The listing builds one solid part. Answer for the finished solid, in the listing's coordinates (mm). Face numbers are marked on the shaded views. A direction names the side the tool comes from. Round coordinates to 2 decimals unless told otherwise and drop trailing zeros. Write each loop counter-clockwise with the first axis right and the second up, starting at its lowest first coordinate (ties: lowest second). Pieces come first, ordered by that corner, then holes. Notation, with made-up numbers: M -9,46 L 29,46 A12 ccw 29,68 Z; hole C -34.75,-31 d8. An arc over 180 degrees is marked long. Put each result on its own line as item: value. Start each with the question number.
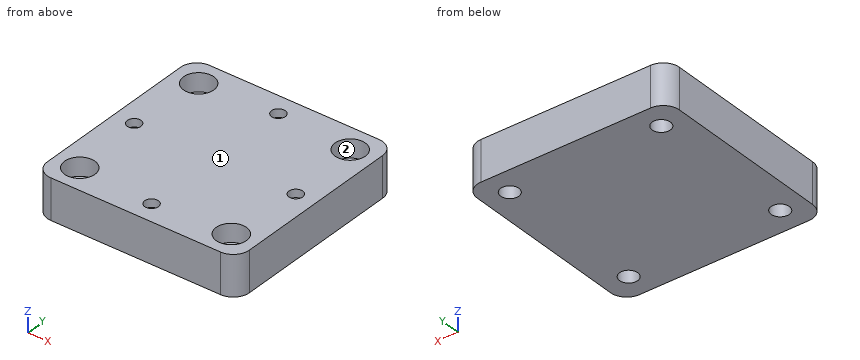
Autodesk Fusion 360 part; units mm, degrees
sketch "Sketch1" plane through (0, 0, 0) normal (0, 0, 1) x (1, 0, 0)
  line L0 (0, 0) -> (-50, 0)
  line L1 (-50, 0) -> (-50, 50)
  line L2 (-50, 50) -> (0, 50)
  line L3 (0, 50) -> (0, 0)
  dimension "d1" = 50
  dimension "d2" = 50
extrude "Extrude1" add sketch "Sketch1" along normal blind 10
sketch "Sketch2" plane through (0, 0, 10) normal (0, 0, 1) x (-1, 0, 0)
  line L0 (0, -50) -> (50, -50)
  line L1 (50, -50) -> (50, 0)
  line L2 (50, 0) -> (0, 0)
  line L3 (0, 0) -> (0, -50)
  line L4 (50, 0) -> (43.75, 0)
  line L5 (43.75, 0) -> (43.75, -6.25)
  line L6 (43.75, -6.25) -> (50, -6.25)
  line L7 (50, -6.25) -> (50, 0)
  line L8 (50, -50) -> (43.75, -50)
  line L9 (43.75, -50) -> (43.75, -43.75)
  line L10 (43.75, -43.75) -> (50, -43.75)
  line L11 (50, -43.75) -> (50, -50)
  line L12 (0, -50) -> (6.25, -50)
  line L13 (6.25, -50) -> (6.25, -43.75)
  line L14 (6.25, -43.75) -> (0, -43.75)
  line L15 (0, -43.75) -> (0, -50)
  line L16 (0, 0) -> (6.25, 0)
  line L17 (6.25, 0) -> (6.25, -6.25)
  line L18 (6.25, -6.25) -> (0, -6.25)
  line L19 (0, -6.25) -> (0, 0)
  circle A0 centre (43.75, -43.75) radius 3.75
  circle A1 centre (6.25, -43.75) radius 3.75
  circle A2 centre (43.75, -6.25) radius 3.75
  circle A3 centre (6.25, -6.25) radius 3.75
  dimension "d5" = 6.25
  dimension "d6" = 6.25
  dimension "d7" = 6.25
  dimension "d8" = 6.25
  dimension "d9" = 6.25
  dimension "d10" = 6.25
  dimension "d11" = 6.25
  dimension "d12" = 6.25
  dimension "d13" = 7.5
  dimension "d14" = 7.5
  dimension "d15" = 7.5
  dimension "d16" = 7.5
extrude "Extrude2" cut sketch "Sketch2" against normal blind 4.5 contours L13 L14 A1 | L13 L14 A1 | L9 L10 A0 | L9 L10 A0 | L17 L18 A3 | L17 L18 A3 | L5 L6 A2 | L5 L6 A2
sketch "Sketch3" plane through (0, 0, 5.5) normal (0, 0, 1) x (-1, 0, 0)
  circle A0 centre (43.75, -43.75) radius 3.75
  circle A1 centre (43.75, -43.75) radius 2.25
  dimension "d19" = 4.5
extrude "Extrude3" cut sketch "Sketch3" against normal blind 10 contours A1
sketch "Sketch4" plane through (0, 0, 5.5) normal (0, 0, 1) x (-1, 0, 0)
  circle A0 centre (6.25, -43.75) radius 3.75
  circle A1 centre (6.25, -43.75) radius 2.25
  dimension "d22" = 4.5
extrude "Extrude4" cut sketch "Sketch4" against normal blind 10 contours A1
sketch "Sketch5" plane through (0, 0, 5.5) normal (0, 0, 1) x (-1, 0, 0)
  circle A0 centre (43.75, -6.25) radius 3.75
  circle A1 centre (43.75, -6.25) radius 2.25
  dimension "d25" = 4.5
extrude "Extrude5" cut sketch "Sketch5" against normal blind 10 contours A1
sketch "Sketch6" plane through (0, 0, 5.5) normal (0, 0, 1) x (-1, 0, 0)
  circle A0 centre (6.25, -6.25) radius 3.75
  circle A1 centre (6.25, -6.25) radius 2.25
  dimension "d28" = 4.5
extrude "Extrude6" cut sketch "Sketch6" against normal blind 10 contours A1
sketch "Sketch7" plane through (0, 0, 10) normal (0, 0, 1) x (-1, 0, 0)
  circle A0 centre (6.25, -43.75) radius 3.75
  circle A1 centre (6.25, -6.25) radius 3.75
  circle A2 centre (43.75, -43.75) radius 3.75
  circle A3 centre (43.75, -6.25) radius 3.75
  line L0 (0, -50) -> (50, -50)
  line L1 (50, -50) -> (50, 0)
  line L2 (50, 0) -> (0, 0)
  line L3 (0, 0) -> (0, -50)
  line L4 (50, 0) -> (37.5, 0)
  line L5 (37.5, 0) -> (37.5, -12.5)
  line L6 (37.5, -12.5) -> (50, -12.5)
  line L7 (50, -12.5) -> (50, 0)
  line L8 (50, -50) -> (37.5, -50)
  line L9 (37.5, -50) -> (37.5, -37.5)
  line L10 (37.5, -37.5) -> (50, -37.5)
  line L11 (50, -37.5) -> (50, -50)
  line L12 (0, -50) -> (12.5, -50)
  line L13 (12.5, -50) -> (12.5, -37.5)
  line L14 (12.5, -37.5) -> (0, -37.5)
  line L15 (0, -37.5) -> (0, -50)
  line L16 (0, 0) -> (12.5, 0)
  line L17 (12.5, 0) -> (12.5, -12.5)
  line L18 (12.5, -12.5) -> (0, -12.5)
  line L19 (0, -12.5) -> (0, 0)
  line L20 (37.5, -12.5) -> (35.5, -12.5)
  line L21 (35.5, -12.5) -> (35.5, -14.5)
  line L22 (35.5, -14.5) -> (37.5, -14.5)
  line L23 (37.5, -14.5) -> (37.5, -12.5)
  line L24 (37.5, -37.5) -> (35.5, -37.5)
  line L25 (35.5, -37.5) -> (35.5, -35.5)
  line L26 (35.5, -35.5) -> (37.5, -35.5)
  line L27 (37.5, -35.5) -> (37.5, -37.5)
  line L28 (12.5, -37.5) -> (14.5, -37.5)
  line L29 (14.5, -37.5) -> (14.5, -35.5)
  line L30 (14.5, -35.5) -> (12.5, -35.5)
  line L31 (12.5, -35.5) -> (12.5, -37.5)
  line L32 (12.5, -12.5) -> (14.5, -12.5)
  line L33 (14.5, -12.5) -> (14.5, -14.5)
  line L34 (14.5, -14.5) -> (12.5, -14.5)
  line L35 (12.5, -14.5) -> (12.5, -12.5)
  dimension "d31" = 12.5
  dimension "d32" = 12.5
  dimension "d33" = 12.5
  dimension "d34" = 12.5
  dimension "d35" = 12.5
  dimension "d36" = 12.5
  dimension "d37" = 12.5
  dimension "d38" = 12.5
  dimension "d39" = 2
  dimension "d40" = 2
  dimension "d41" = 2
  dimension "d42" = 2
  dimension "d43" = 2
  dimension "d44" = 2
  dimension "d45" = 2
  dimension "d46" = 2
extrude "Extrude7" add sketch "Sketch7" along normal blind 2 contours L24 L25 L26 L27 | L20 L21 L22 L23 | L32 L33 L34 L35 | L28 L29 L30 L31
extrude "Extrude8" cut 4 faces at (-13.1667, 36.1667, 12) (-13.1667, 13.1667, 12) (-36.1667, 13.1667, 12) (-36.8333, 36.8333, 12) along direction (0, 0, -1) blind 2
fillet "Fillet1" radius 4 1 edges at (0, 50, 5)
fillet "Fillet2" radius 4 1 edges at (0, 0, 5)
fillet "Fillet3" radius 4 1 edges at (-50, 50, 5)
fillet "Fillet4" radius 4 1 edges at (-50, 0, 5)
sketch "Sketch8" plane through (0, 0, 10) normal (0, 0, 1) x (-1, 0, 0)
  circle A0 centre (6.25, -43.75) radius 3.75
  circle A1 centre (6.25, -6.25) radius 3.75
  circle A2 centre (43.75, -43.75) radius 3.75
  circle A3 centre (43.75, -6.25) radius 3.75
  arc A4 (50, -4) -> (46, 0) centre (46, -4) ccw
  line L0 (46, 0) -> (4, 0)
  arc A5 (4, 0) -> (0, -4) centre (4, -4) ccw
  line L1 (0, -4) -> (0, -46)
  arc A6 (0, -46) -> (4, -50) centre (4, -46) ccw
  line L2 (4, -50) -> (46, -50)
  arc A7 (46, -50) -> (50, -46) centre (46, -46) ccw
  line L3 (50, -46) -> (50, -4)
  line L4 (0, 0) -> (5, 0)
  line L5 (5, 0) -> (5, -5)
  line L6 (5, -5) -> (0, -5)
  line L7 (0, -5) -> (0, 0)
  line L8 (5, -5) -> (45, -5)
  line L9 (45, -5) -> (45, -45)
  line L10 (45, -45) -> (5, -45)
  line L11 (5, -45) -> (5, -5)
  circle A8 centre (25, -45) radius 1.6
  circle A9 centre (45, -25) radius 1.6
  circle A10 centre (25, -5) radius 1.6
  circle A11 centre (5, -25) radius 1.6
  dimension "d59" = 5
  dimension "d60" = 5
  dimension "d61" = 40
  dimension "d62" = 40
  dimension "d63" = 3.2
  dimension "d64" = 3.2
  dimension "d65" = 3.2
  dimension "d66" = 3.2
extrude "Extrude9" cut sketch "Sketch8" against normal blind 2 contours L11 A11 | L11 A11 | L10 A8 | L10 A8 | L9 A9 | L9 A9 | L8 A10 | L8 A10
sketch "Sketch9" plane through (0, 0, 10) normal (0, 0, 1) x (-1, 0, 0)
  circle A0 centre (25, -45) radius 1.6
  circle A1 centre (5, -25) radius 1.6
  circle A2 centre (45, -25) radius 1.6
  circle A3 centre (25, -5) radius 1.6
  circle A4 centre (6.25, -43.75) radius 3.75
  circle A5 centre (6.25, -6.25) radius 3.75
  circle A6 centre (43.75, -43.75) radius 3.75
  circle A7 centre (43.75, -6.25) radius 3.75
  arc A8 (50, -4) -> (46, 0) centre (46, -4) ccw
  line L0 (46, 0) -> (4, 0)
  arc A9 (4, 0) -> (0, -4) centre (4, -4) ccw
  line L1 (0, -4) -> (0, -46)
  arc A10 (0, -46) -> (4, -50) centre (4, -46) ccw
  line L2 (4, -50) -> (46, -50)
  arc A11 (46, -50) -> (50, -46) centre (46, -46) ccw
  line L3 (50, -46) -> (50, -4)
  circle A12 centre (25, -5) radius 1.7
  dimension "d69" = 3.4
extrude "Extrude10" cut sketch "Sketch9" against normal blind 2 contours A12
sketch "Sketch10" plane through (0, 0, 10) normal (0, 0, 1) x (-1, 0, 0)
  circle A0 centre (25, -5) radius 1.7
  circle A1 centre (25, -45) radius 1.6
  circle A2 centre (5, -25) radius 1.6
  circle A3 centre (45, -25) radius 1.6
  circle A4 centre (6.25, -43.75) radius 3.75
  circle A5 centre (6.25, -6.25) radius 3.75
  circle A6 centre (43.75, -43.75) radius 3.75
  circle A7 centre (43.75, -6.25) radius 3.75
  arc A8 (50, -4) -> (46, 0) centre (46, -4) ccw
  line L0 (46, 0) -> (4, 0)
  arc A9 (4, 0) -> (0, -4) centre (4, -4) ccw
  line L1 (0, -4) -> (0, -46)
  arc A10 (0, -46) -> (4, -50) centre (4, -46) ccw
  line L2 (4, -50) -> (46, -50)
  arc A11 (46, -50) -> (50, -46) centre (46, -46) ccw
  line L3 (50, -46) -> (50, -4)
  circle A12 centre (45, -25) radius 1.7
  dimension "d72" = 3.4
extrude "Extrude11" cut sketch "Sketch10" against normal blind 2 contours A12
sketch "Sketch11" plane through (0, 0, 10) normal (0, 0, 1) x (-1, 0, 0)
  circle A0 centre (45, -25) radius 1.7
  circle A1 centre (25, -5) radius 1.7
  circle A2 centre (25, -45) radius 1.6
  circle A3 centre (5, -25) radius 1.6
  circle A4 centre (6.25, -43.75) radius 3.75
  circle A5 centre (6.25, -6.25) radius 3.75
  circle A6 centre (43.75, -43.75) radius 3.75
  circle A7 centre (43.75, -6.25) radius 3.75
  arc A8 (50, -4) -> (46, 0) centre (46, -4) ccw
  line L0 (46, 0) -> (4, 0)
  arc A9 (4, 0) -> (0, -4) centre (4, -4) ccw
  line L1 (0, -4) -> (0, -46)
  arc A10 (0, -46) -> (4, -50) centre (4, -46) ccw
  line L2 (4, -50) -> (46, -50)
  arc A11 (46, -50) -> (50, -46) centre (46, -46) ccw
  line L3 (50, -46) -> (50, -4)
  circle A12 centre (5, -25) radius 1.7
  dimension "d75" = 3.4
extrude "Extrude12" cut sketch "Sketch11" against normal blind 2 contours A12
sketch "Sketch12" plane through (0, 0, 10) normal (0, 0, 1) x (-1, 0, 0)
  circle A0 centre (5, -25) radius 1.7
  circle A1 centre (45, -25) radius 1.7
  circle A2 centre (25, -5) radius 1.7
  circle A3 centre (25, -45) radius 1.6
  circle A4 centre (6.25, -43.75) radius 3.75
  circle A5 centre (6.25, -6.25) radius 3.75
  circle A6 centre (43.75, -43.75) radius 3.75
  circle A7 centre (43.75, -6.25) radius 3.75
  arc A8 (50, -4) -> (46, 0) centre (46, -4) ccw
  line L0 (46, 0) -> (4, 0)
  arc A9 (4, 0) -> (0, -4) centre (4, -4) ccw
  line L1 (0, -4) -> (0, -46)
  arc A10 (0, -46) -> (4, -50) centre (4, -46) ccw
  line L2 (4, -50) -> (46, -50)
  arc A11 (46, -50) -> (50, -46) centre (46, -46) ccw
  line L3 (50, -46) -> (50, -4)
  circle A12 centre (25, -45) radius 1.7
  dimension "d78" = 3.4
extrude "Extrude13" cut sketch "Sketch12" against normal blind 2 contours A12
Item 1: Flat-ended cylindrical pins translate along their axes: pin 1 (2.5 mm diameter, centred on x = -6.25, y = 43.75, fed in from +Z); pin 2 (1.7 mm diameter, centred on x = -25, y = 5.5, fed in from +Z); pin 3 (7 mm diameter, centred on x = -6.25, y = 6.25, fed in from +Z). Find the tip coordinate at first contact, or state that the pin passes through.
Item 2: Which of the six approach directions +Z, -Z, +X, -X, +Y, -Y give full straight-line access (tool end or side, diameter ignored) to the marked faces 1 and 2?
Item 3: Section B-B (x = -45) is taken. Give the vertices of the cut face in (y, z), and give its area (3 significant figures).
Item 4: Consider line 1 along Y through (x, z) = (-25, 9); line 2 along X through (y, z) = (25, 9.3); line 3 along Y through (x, z) = (-43.75, 1.7). Determine where each line is inside the solid, lowest interval first. Write a range as [from, to].
Item 5: Section A-A (z = 6.5) is taken. Give the vertices of the cut face in (x, y).
Item 6: Section C-C (y = 45) is taken. Give the vertices of the cut face in (x, z), and give its area (3 significant figures).
Item 7: Section D-D (x = -25) is taken. Give the vertices of the cut face in (y, z).
Output values:
1. pin 1: passes through
1. pin 2: stops at z = 8
1. pin 3: stops at z = 5.5
2. face 1: +Z, +X, -X, +Y, -Y
2. face 2: +Z
3. outline: M 0,0 L 4.38,0 L 4.38,5.5 L 2.71,5.5 L 2.71,10 L 0,10 Z; M 8.12,0 L 41.88,0 L 41.88,5.5 L 40.21,5.5 L 40.21,10 L 26.7,10 L 26.7,8 L 23.3,8 L 23.3,10 L 9.79,10 L 9.79,5.5 L 8.12,5.5 Z; M 45.62,0 L 50,0 L 50,10 L 47.29,10 L 47.29,5.5 L 45.62,5.5 Z
3. area: 388 mm^2
4. line 1: y = [0, 3.3], [6.7, 43.3], [46.7, 50]
4. line 2: x = [-50, -46.7], [-43.3, -6.7], [-3.3, 0]
4. line 3: y = [0, 4], [8.5, 41.5], [46, 50]
5. outline: M -50,4 A4 ccw -46,0 L -4,0 A4 ccw 0,4 L 0,46 A4 ccw -4,50 L -46,50 A4 ccw -50,46 Z; hole C -43.75,6.25 d7.5; hole C -43.75,43.75 d7.5; hole C -6.25,6.25 d7.5; hole C -6.25,43.75 d7.5
6. outline: M -50,0 L -45.62,0 L -45.62,5.5 L -47.29,5.5 L -47.29,10 L -50,10 Z; M -41.88,0 L -8.12,0 L -8.12,5.5 L -9.79,5.5 L -9.79,10 L -23.3,10 L -23.3,8 L -26.7,8 L -26.7,10 L -40.21,10 L -40.21,5.5 L -41.88,5.5 Z; M -4.38,0 L 0,0 L 0,10 L -2.71,10 L -2.71,5.5 L -4.38,5.5 Z
6. area: 388 mm^2
7. outline: M 0,0 L 50,0 L 50,10 L 46.7,10 L 46.7,8 L 43.3,8 L 43.3,10 L 6.7,10 L 6.7,8 L 3.3,8 L 3.3,10 L 0,10 Z
